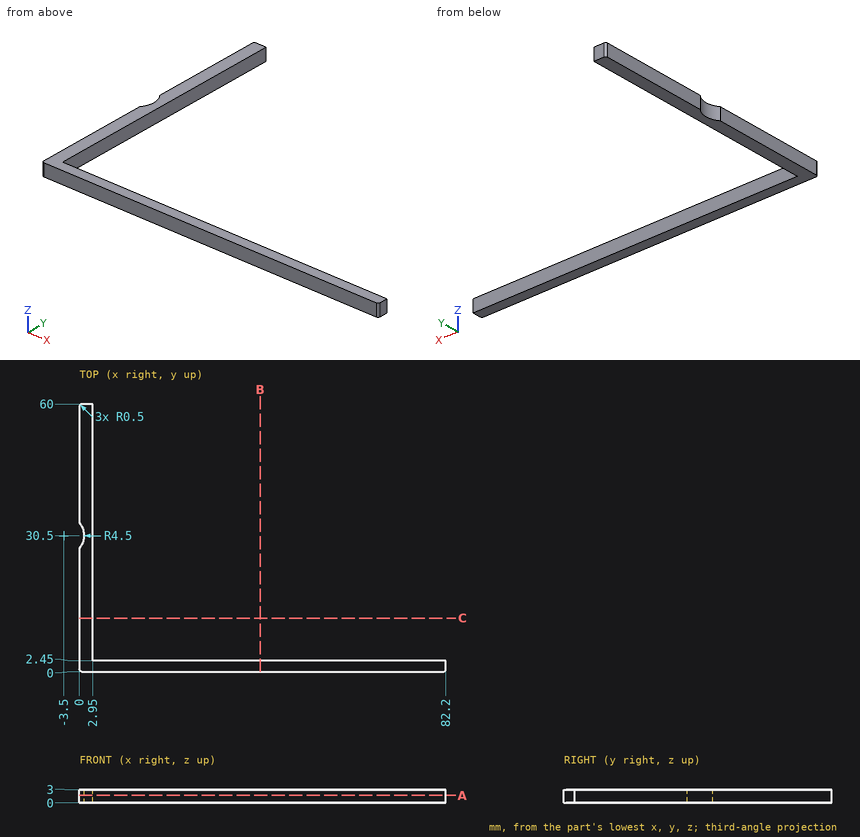
Verification items for this drawing (mm, ordinates from the low corner). Give positions to 0.01 mm unless a question says otherwise; leave off trailing zeros. Write each loop counter-clockwise with the first axis right and the second up, starting at its lowest first coordinate (ties: lowest second). Pieces come first, ordered by that corner, then holes. Notation, with made-up numbers: (-3, -5.75) -> (21, -5.75) arc R32 ccw to (21, 23.25) -> close; hole circle Ø4 at (85.25, 27). An arc over 180 degrees is marked (long way). Use CSV: the item, a comma, the result in double quotes. Start each with the question number.
Q1. Cross-section at A-A on z = 1.7. Enter the section's corners in (x, y).
Q2. Depth check by flat-ended pin: P1, Ø0.9, axis at x = 60, z = 1, coming from the +Y side; P2, Ø12, axis at x = 9, y = 15, coming from the +Z side. Enter the tip coordinate at first touch or a pass-through.
Q3. Cross-section at B-B on x = 40.5. Enter the section's corners in (y, z), and give its area (3 significant figures).
Q4. Cross-section at C-C on y = 12. Enter the section's corners in (x, z).
Q5. Scan lines: line 1 along X through (y, z) = (7, 1.9); line 2 along Y through (x, z) = (33, 1.1); line 3 along X through (y, z) = (32.5, 2.7). Record each from-to range of solid material in increasing order.
Working result:
1,outline,"(0, 0.5) arc R0.5 ccw to (0.5, 0) -> (81.7, 0) arc R0.5 ccw to (82.2, 0.5) -> (82.2, 2.45) -> (2.95, 2.45) -> (2.95, 60) -> (0.5, 60) arc R0.5 ccw to (0, 59.5) -> (0, 33.33) arc R4.5 cw to (0, 27.67) -> close"
2,P1,"stops at y = 2.45"
2,P2,"passes through"
3,outline,"(0, 0) -> (2.45, 0) -> (2.45, 3) -> (0, 3) -> close"
3,area,"7.35 mm^2"
4,outline,"(0, 0) -> (2.95, 0) -> (2.95, 3) -> (0, 3) -> close"
5,line 1,"x = 0 to 2.95"
5,line 2,"y = 0 to 2.45"
5,line 3,"x = 0.53 to 2.95"
